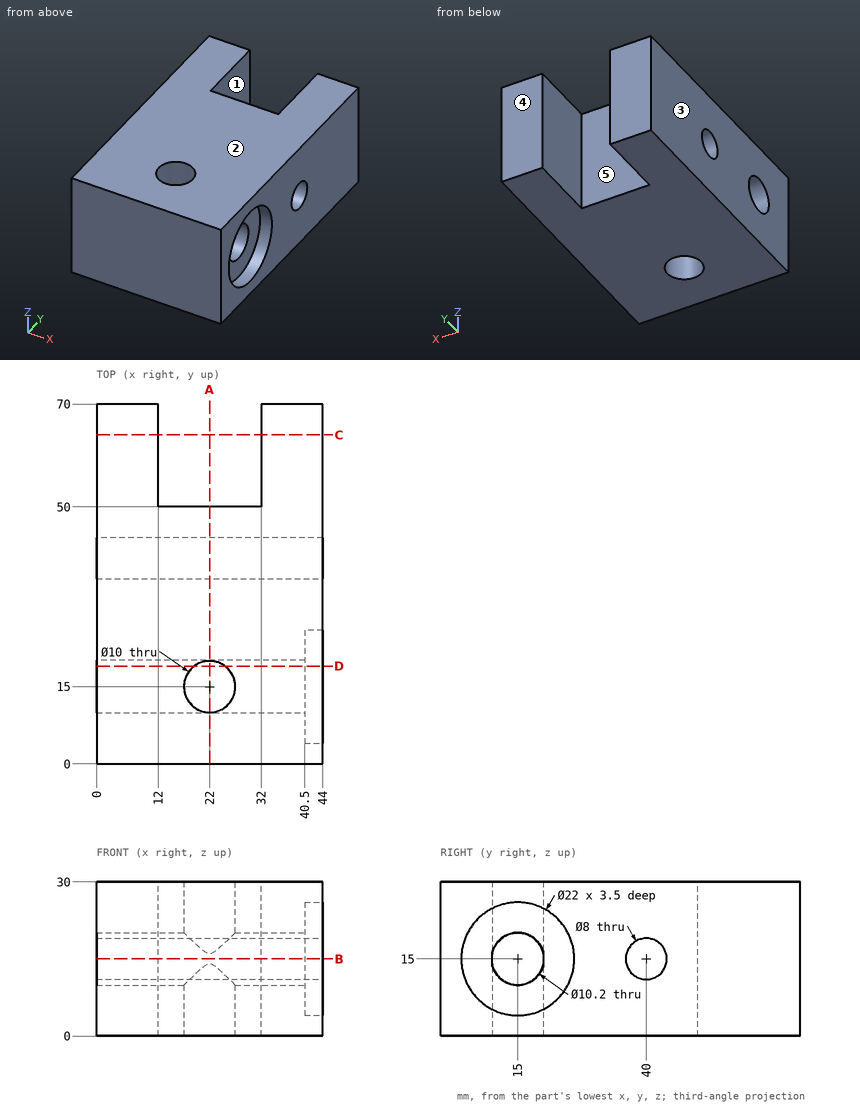
Study the drawing (mm; zero at the part's minimum x, y, z) and answer. A direction names the side the tool comes from. Give positions to 0.01 mm unless a question says otherwise; leave off trailing zeros. Write each loop counter-clockwise with the first axis right and the second up, starting at its lowest first coordinate (ties: lowest second). Pieces come first, ordered by that corner, then holes.
(1) The part is cut by section D-D on y = 19. Write down the section's boundary in (x, z), plus the area to 3 significant figures.
Final values:
outline: (0, 0) - (19, 0) - (19, 11.84) - (0, 11.84) - close; (0, 18.16) - (19, 18.16) - (19, 30) - (0, 30) - close; (25, 0) - (44, 0) - (44, 4.75) - (40.5, 4.75) - (40.5, 11.84) - (25, 11.84) - close; (25, 18.16) - (40.5, 18.16) - (40.5, 25.25) - (44, 25.25) - (44, 30) - (25, 30) - close
area: 850 mm2
(2) The mould has two halves that part along X. Classify the marked faces 3, 4 and 5: pulls with the +X half, pulls with the -X half, needs draft (parallel to the pull), parting line crosses it, or undercut.
Final values:
face 3: pulls with the -X half
face 4: needs draft
face 5: undercut
(3) The part is cut by section A-A on x = 22. Write down the section's boundary in (y, z).
Final values:
outline: (0, 0) - (10, 0) - (10, 14) arc R5.1 cw to (10, 16) - (10, 30) - (0, 30) - close; (20, 0) - (50, 0) - (50, 30) - (20, 30) - (20, 16) arc R5.1 cw to (20, 14) - close; hole circle Ø8 at (40, 15)
(4) Straight lines are drawn through the part: line 1 (X direction, y = 15, z = 6); line 2 (Y direction, x = 22, z = 27.25); line 3 (X direction, y = 15, z = 27.25). For each, find the intervals that lie inside material, in ascending order.
Final values:
line 1: x = 0 to 17, 27 to 40.5
line 2: y = 0 to 10, 20 to 50
line 3: x = 0 to 17, 27 to 44
(5) Flat-ended cylindrical pins translate along their axes: pin 1 Ø5 at (x, z) = (5.5, 11.5) entering from -Y; pin 2 Ø11.5 at (y, z) = (15, 15) entering from +X; pin 3 Ø6 at (x, z) = (23, 12) entering from +Y. Find the tip coordinate at first contact, or state that the pin passes through.
Final values:
pin 1: stops at y = 0
pin 2: stops at x = 40.5
pin 3: stops at y = 50
(6) The part is cut by section C-C on y = 64. Write down the section's boundary in (x, z).
Final values:
outline: (0, 0) - (12, 0) - (12, 30) - (0, 30) - close; (32, 0) - (44, 0) - (44, 30) - (32, 30) - close
(7) Which of the six approach directions +Z, -Z, +X, -X, +Y, -Y give full straight-line access (tool end or side, diameter ignored) to the marked faces 1 and 2?
Final values:
face 1: +Z, -Z, +Y
face 2: +Z, +X, -X, +Y, -Y
(8) The part is cut by section B-B on z = 15. Write down the section's boundary in (x, y).
Final values:
outline: (0, 0) - (44, 0) - (44, 4) - (40.5, 4) - (40.5, 9.9) - (0, 9.9) - close; (0, 20.1) - (40.5, 20.1) - (40.5, 26) - (44, 26) - (44, 36) - (0, 36) - close; (0, 44) - (44, 44) - (44, 70) - (32, 70) - (32, 50) - (12, 50) - (12, 70) - (0, 70) - close
